from build123d import *

# Parameters (mm, degrees)
SKETCH1_W           = 88.9
SKETCH1_H           = 63.5
BOSS_EXTRUDE1_DEPTH = 19.05
CUT_EXTRUDE1_DEPTH  = 97.302518139
SKETCH7_W           = 5.334
SKETCH7_H           = 35.71875
SKETCH7_W_2         = 38.1
SKETCH7_H_2         = 44.45
CUT_EXTRUDE4_DEPTH  = 67.599361859
SKETCH4_R           = 6.985
CUT_EXTRUDE3_DEPTH  = 75.865395878
SKETCH6_R           = 2.413
SKETCH5_R           = 5.08
CIRPATTERN1_COUNT   = 4
FILLET1_R           = 3.175


with BuildPart() as part:
    # Sketch1 → Boss-Extrude1 (new, symmetric)
    with BuildSketch(Plane(origin=(0, 0, 0), x_dir=(1, 0, 0), z_dir=(0, 1, 0))):
        Rectangle(SKETCH1_W, SKETCH1_H)
    extrude(amount=BOSS_EXTRUDE1_DEPTH, both=True)

    # Sketch3 → Cut-Extrude1 (cut, through all)
    with BuildSketch(Plane(origin=(44.45, 0, 0), x_dir=(0, 0, -1), z_dir=(1, 0, 0))):
        Polygon((-31.75, 10.31875), (-31.75, -10.31875), (-28.575, -10.31875), (-28.575, -16.66875), (-21.43125, -16.66875), (-21.43125, -10.31875), (18.653125, -10.31875), (18.653125, -7.14375), (21.828125, -7.14375), (21.828125, -10.31875), (25.4, -10.31875), (25.4, 10.31875), (21.828125, 10.31875), (21.828125, 7.14375), (18.653125, 7.14375), (18.653125, 10.31875), (-21.43125, 10.31875), (-21.43125, 16.66875), (-28.575, 16.66875), (-28.575, 10.31875), align=None)
    extrude(amount=-CUT_EXTRUDE1_DEPTH, mode=Mode.SUBTRACT)

    # Sketch7 → Cut-Extrude4 (cut, through all)
    with BuildSketch(Plane(origin=(0, 19.05, 0), x_dir=(1, 0, 0), z_dir=(0, 1, 0))):
        with Locations((-32.54375, -1.190625)):
            Rectangle(SKETCH7_W, SKETCH7_H)
        with Locations((32.54375, -1.190625)):
            Rectangle(SKETCH7_W, SKETCH7_H)
        with Locations((0, 3.175)):
            Rectangle(SKETCH7_W_2, SKETCH7_H_2)
    extrude(amount=-CUT_EXTRUDE4_DEPTH, mode=Mode.SUBTRACT)

    # Sketch4 → Cut-Extrude3 (cut, through all)
    with BuildSketch(Plane.XY.offset(-25.4)):
        Circle(SKETCH4_R)
        with BuildLine():
            ThreePointArc((-5.842, 8.255), (-9.961248663, 9.961248663), (-8.255, 5.842))
            Line((-8.255, 5.842), (-8.255, 8.255))
            Line((-8.255, 8.255), (-5.842, 8.255))
        make_face()
        with BuildLine():
            Line((-8.255, 8.255), (-8.255, 5.842))
            ThreePointArc((-8.255, 5.842), (-6.548751337, 6.548751337), (-5.842, 8.255))
            Line((-5.842, 8.255), (-8.255, 8.255))
        make_face()
        with BuildLine():
            ThreePointArc((5.842, 8.255), (6.548751337, 6.548751337), (8.255, 5.842))
            Line((8.255, 5.842), (8.255, 8.255))
            Line((8.255, 8.255), (5.842, 8.255))
        make_face()
        with BuildLine():
            Line((8.255, 8.255), (8.255, 5.842))
            ThreePointArc((8.255, 5.842), (9.961248663, 6.548751337), (10.668, 8.255))
            ThreePointArc((10.668, 8.255), (8.255, 10.668), (5.842, 8.255))
            Line((5.842, 8.255), (8.255, 8.255))
        make_face()
        with BuildLine():
            ThreePointArc((8.255, -5.842), (6.548751337, -6.548751337), (5.842, -8.255))
            Line((5.842, -8.255), (8.255, -8.255))
            Line((8.255, -8.255), (8.255, -5.842))
        make_face()
        with BuildLine():
            Line((8.255, -8.255), (5.842, -8.255))
            ThreePointArc((5.842, -8.255), (8.255, -10.668), (10.668, -8.255))
            ThreePointArc((10.668, -8.255), (9.961248663, -6.548751337), (8.255, -5.842))
            Line((8.255, -5.842), (8.255, -8.255))
        make_face()
        with BuildLine():
            ThreePointArc((-8.255, -5.842), (-9.961248663, -9.961248663), (-5.842, -8.255))
            Line((-5.842, -8.255), (-8.255, -8.255))
            Line((-8.255, -8.255), (-8.255, -5.842))
        make_face()
        with BuildLine():
            Line((-8.255, -8.255), (-5.842, -8.255))
            ThreePointArc((-5.842, -8.255), (-6.548751337, -6.548751337), (-8.255, -5.842))
            Line((-8.255, -5.842), (-8.255, -8.255))
        make_face()
    extrude(amount=-CUT_EXTRUDE3_DEPTH, mode=Mode.SUBTRACT)

    # Sketch6 → Cut-Loft2 section 0
    with BuildSketch(Plane.XY.offset(-28.575)):
        with Locations((-8.255, 8.255)):
            Circle(SKETCH6_R)
    # Sketch5 → Cut-Loft2 section 1
    with BuildSketch(Plane.XY.offset(-25.4)):
        with Locations((-8.255, 8.255)):
            Circle(SKETCH5_R)
    cut_loft2 = loft(mode=Mode.SUBTRACT)

    # CirPattern1: Cut-Loft2 ×4 about axis
    cirpattern1_axis = Axis((0, 0, 0), (0, 0, 1))
    for i in range(1, CIRPATTERN1_COUNT):
        add(cut_loft2.rotate(cirpattern1_axis, i * 360 / CIRPATTERN1_COUNT), mode=Mode.SUBTRACT)

    # Fillet1
    fillet1_edges = [part.edges().sort_by_distance(p)[0] for p in [
        (19.05, -14.684375, 19.05),
        (-19.05, -14.684375, 19.05),
        (-19.05, -14.684375, -25.4),
        (19.05, -14.684375, -25.4),
        (-19.05, 14.684375, 19.05),
        (-19.05, 14.684375, -25.4),
        (19.05, 14.684375, -25.4),
        (19.05, 14.684375, 19.05),
    ]]
    fillet(fillet1_edges, radius=FILLET1_R)


solid = part.part
Work out the finished part from the listing and answer in its coordinate system (mm). A direction names the side the tool comes from. Give positions to 0.01 mm unless a question says otherwise; leave off trailing zeros. Loops run counter-clockwise (first coordinate to the right, second up) from the corner with the lowest first, then second, coordinate; pieces in that order, holes last. Notation, with made-up numbers: (82.5, 64) -> (91.5, 64) arc R7 cw to (91.5, 72) -> close; hole circle Ø2 at (24.25, 76). An arc over 180 degrees is marked (long way). Use a Markdown table: item, result. Add a question column.
1. Section B-B on z = 12 is taken. State how many separate pieces and enclosed holes the cut face has, and give its area (3 significant figures).
2. Section C-C on x = 0 is taken. Determine the outline of the cut face in (y, z) (3 decimals), and give its area (3 significant figures).
3. Section D-D on x = 37.5 is taken. Determine the outline of the cut face in (y, z) (3 decimals), and give its area (3 significant figures).
4. Section A-A on y = 0 is taken. Determine the outline of the cut face in (x, z) (3 decimals).
5. Find the intervals of material crossed by probe 1 along X at (y, z) = (16, -2); probe 2 along Z at (x, y) = (-6, 13) (3 decimals); probe 3 along Z at (x, y) = (41, -8.5), in increasing order.
6. Determine the mould class of faces 5 (the conical face through (-5.97, -7.06, -28.38)), 6 (the flat face through (-1, -15, 31.75)) for opening direction X: released by +X, released by -X, zero draft, split by the parting line, or undercut.
7. For faces 1 (the conical face through (-8.81, 5.74, -28.38)), 2 (the flat face through (1, 10.319, 30)), 3 (the flat face through (-33, -15, 19.05)), 4 (the flat face through (-32, -9, -21.828)), determine the directions among +Z, -Z, +X, -X, +Y, -Y from which every point of the face is accessible in a straight line to the end or side of a thin tool.
8. Flat-ended cylindrical pins translate along their axes: pin 1 Ø1 at (x, y) = (1.5, 9) entering from +Z; pin 2 Ø18 at (x, y) = (0, 0) entering from -Z; pin 3 Ø1 at (x, y) = (-31, -8.5) entering from +Z. Find the tip coordinate at first contact, or state that the pin passes through.
Results below:
| question | item | result |
|---|---|---|
| 1 | separate pieces | 8 |
| 1 | enclosed holes | 0 |
| 1 | area | 701 mm^2 |
| 2 | outline | (-19.05, -31.75) -> (-6.985, -31.75) -> (-6.985, -25.4) -> (-19.05, -25.4) -> close; (-19.05, 19.05) -> (-10.319, 19.05) -> (-10.319, 21.431) -> (-16.669, 21.431) -> (-16.669, 28.575) -> (-10.319, 28.575) -> (-10.319, 31.75) -> (-19.05, 31.75) -> close; (6.985, -31.75) -> (19.05, -31.75) -> (19.05, -25.4) -> (6.985, -25.4) -> close; (10.319, 19.05) -> (19.05, 19.05) -> (19.05, 31.75) -> (10.319, 31.75) -> (10.319, 28.575) -> (16.669, 28.575) -> (16.669, 21.431) -> (10.319, 21.431) -> close |
| 2 | area | 284 mm^2 |
| 3 | outline | (-19.05, -31.75) -> (19.05, -31.75) -> (19.05, 31.75) -> (10.319, 31.75) -> (10.319, 28.575) -> (16.669, 28.575) -> (16.669, 21.431) -> (10.319, 21.431) -> (10.319, -18.653) -> (7.144, -18.653) -> (7.144, -21.828) -> (10.319, -21.828) -> (10.319, -25.4) -> (-10.319, -25.4) -> (-10.319, -21.828) -> (-7.144, -21.828) -> (-7.144, -18.653) -> (-10.319, -18.653) -> (-10.319, 21.431) -> (-16.669, 21.431) -> (-16.669, 28.575) -> (-10.319, 28.575) -> (-10.319, 31.75) -> (-19.05, 31.75) -> close |
| 3 | area | 1,170 mm^2 |
| 4 | outline | (-44.45, -31.75) -> (-6.985, -31.75) -> (-6.985, -25.4) -> (-44.45, -25.4) -> close; (6.985, -31.75) -> (44.45, -31.75) -> (44.45, -25.4) -> (6.985, -25.4) -> close |
| 5 | probe 1 | x = -44.45 to -35.21, -29.88 to -19.05, 19.05 to 29.88, 35.21 to 44.45 |
| 5 | probe 2 | z = -31.75 to -25.4, 19.05 to 21.431, 28.575 to 31.75 |
| 5 | probe 3 | z = -31.75 to -25.4, -21.83 to -18.65 |
| 6 | face 5 | undercut |
| 6 | face 6 | zero draft |
| 7 | face 1 | none |
| 7 | face 2 | +Z, +X, -X |
| 7 | face 3 | +Y, -Y |
| 7 | face 4 | +X, -X |
| 8 | pin 1 | stops at z = -25.4 |
| 8 | pin 2 | stops at z = -31.75 |
| 8 | pin 3 | stops at z = -18.65 |
